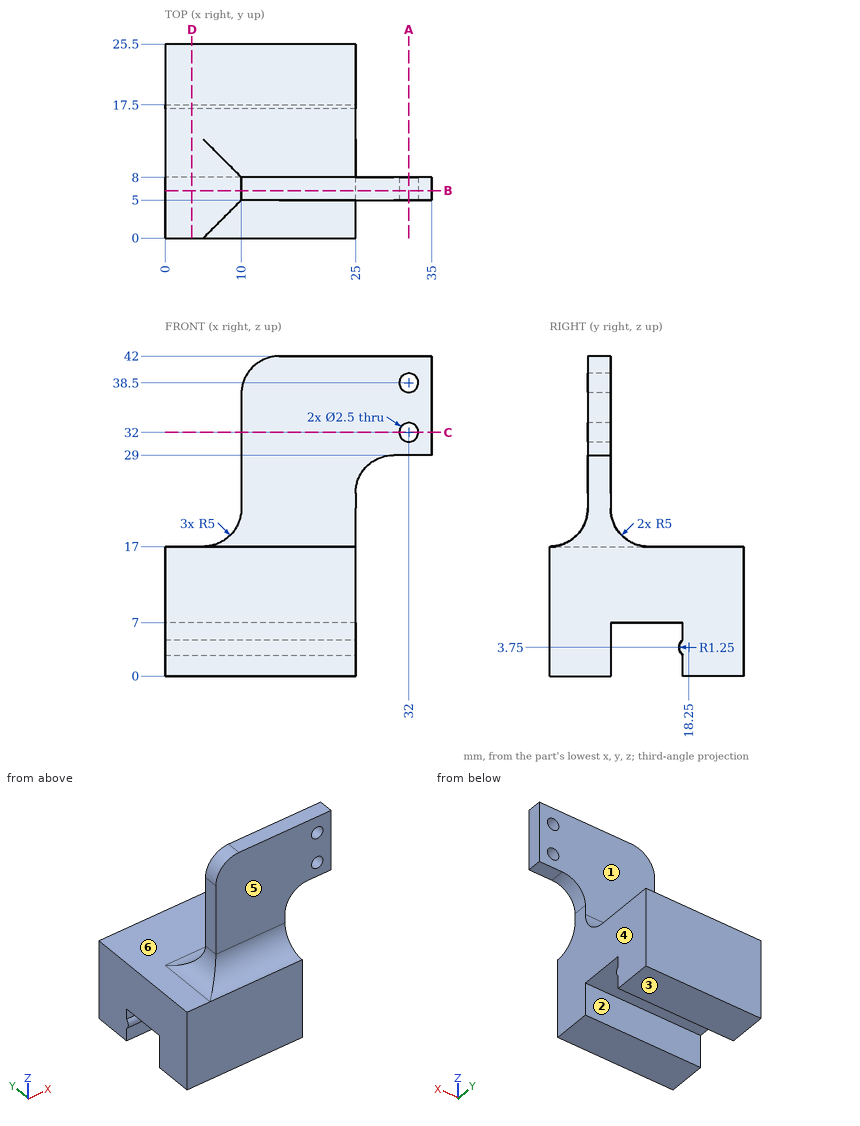
Input: dimensioned drawing with shaded views. Units: mm. Origin: part minimum x, y, z. A direction names the side the tool comes from. Round coordinates to 2 decimals unless told otherwise and drop trailing zeros. Loops run counter-clockwise (first coordinate to the right, second up) from the corner with the lowest first, then second, coordinate; pieces in that order, holes last. Notation, with made-up numbers: M 40.25,35 L 67.25,35 A29 cw 67.25,64 Z; hole C -36,69.5 d7. An arc over 180 degrees is marked long. One line per question, with ' | ' between items.
(1) Cut plane B-B on y = 6.25. Return the cut outline in (x, z).
Check result:
outline: M 0,0 L 25,0 L 25,24 A5 cw 30,29 L 35,29 L 35,42 L 15,42 A5 ccw 10,37 L 10,22 A5 cw 5,17 L 0,17 Z; hole C 32,32 d2.5; hole C 32,38.5 d2.5
(2) Contact query for flat-ended pins moving along their axis: P1, Ø10, axis at x = 27, z = 33, coming from the +Y side; P2, Ø12, axis at y = 10.5, z = 32, coming from the -X side; P3, Ø1.5, axis at x = 32, z = 38.5, coming from the +Y side; P4, Ø1.5, axis at x = 21, z = 32, coming from the -Y side. Output: stop coordinate, or through.
Check result:
P1: stops at y = 8 | P2: stops at x = 10 | P3: passes through | P4: stops at y = 5
(3) Material intervals for line 1 along X through (y, z) = (7.45, 32); line 2 along X through (y, z) = (5.75, 3); line 3 along X through (y, z) = (6.2, 38.5), sorted ascending. Write a range as from..to.
Check result:
line 1: x = 10..30.75, 33.25..35 | line 2: x = 0..25 | line 3: x = 10.23..30.75, 33.25..35
(4) Cut plane D-D on x = 3.5. Return the cut outline in (y, z), plus the area to 3 significant figures.
Check result:
outline: M 0,0 L 8,0 L 8,7 L 17.5,7 L 17.5,4.75 A1.25 ccw 17.5,2.75 L 17.5,0 L 25.5,0 L 25.5,17 L 0,17 Z | area: 368 mm2
(5) Cut plane A-A on x = 32. Return the cut outline in (y, z).
Check result:
outline: M 5,29 L 8,29 L 8,30.75 L 5,30.75 Z; M 5,33.25 L 8,33.25 L 8,37.25 L 5,37.25 Z; M 5,39.75 L 8,39.75 L 8,42 L 5,42 Z
(6) Pull-direction query (Y, two-part tool) for the marked faces 1, 2 and 3; classes: +Y half, -Y half, draft (parallel to the pull), parting line (faces both ways), or undercut.
Check result:
face 1: +Y half | face 2: undercut | face 3: draft
(7) Cut plane C-C on z = 32. Return the cut outline in (x, y).
Check result:
outline: M 10,5 L 30.75,5 L 30.75,8 L 10,8 Z; M 33.25,5 L 35,5 L 35,8 L 33.25,8 Z
(8) Access query for the marked faces 4, 5 and 6. Directions: +Z, -Z, +X, -X, +Y, -Y. A direction counts if a zero-diameter tool reaches every point of the face in a straight line with its end or side. Return the directions, or none.
Check result:
face 4: -Z, +X, +Y, -Y | face 5: +Z, +X, -X, -Y | face 6: +Z, -X, +Y
